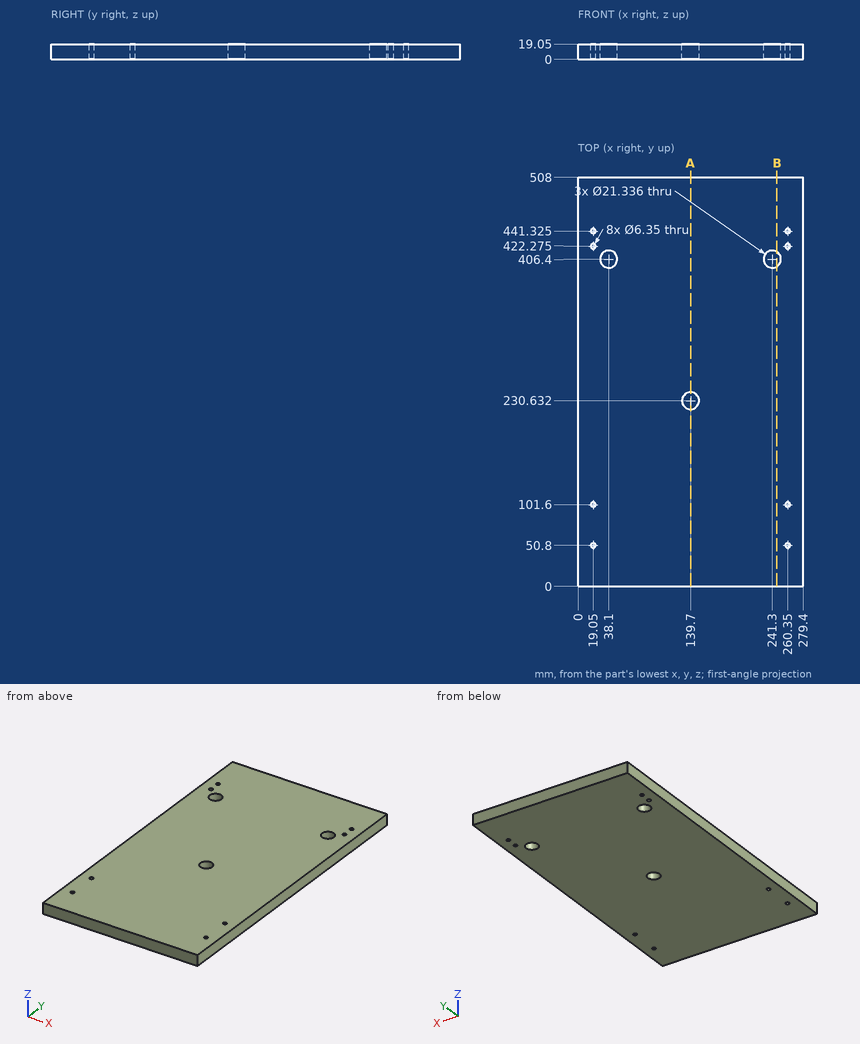
Part print with two shaded views. Sizes in mm from the minimum x, y, z corner. Coordinates: 2 decimals unless noted, no trailing zeros. Write each loop counter-clockwise with the first axis right and the second up, starting at its lowest first coordinate (ties: lowest second). Pieces come first, ordered by that corner, then holes. Notation, with made-up numbers: M 75,15.5 L 108,15.5 A21 ccw 108,51.5 Z; hole C -37,2 d4. An arc over 180 degrees is marked long. Return JSON: item names as keys, results as strings.
Item 1: Slice it at B-B, the plane x = 247. Write the cut outline in (y, z), and give its area (3 significant figures).
Findings below:
{"outline": "M 0,0 L 397.38,0 L 397.38,19.05 L 0,19.05 Z; M 415.42,0 L 508,0 L 508,19.05 L 415.42,19.05 Z", "area": "9,330 mm2"}
Item 2: Slice it at A-A, the plane x = 139.7. Write the cut outline in (y, z), and give its area (3 significant figures).
Findings below:
{"outline": "M 0,0 L 219.96,0 L 219.96,19.05 L 0,19.05 Z; M 241.3,0 L 508,0 L 508,19.05 L 241.3,19.05 Z", "area": "9,270 mm2"}
Item 3: Drop a flat-ended pin along its axis: pin 1 Ø5 at (x, y) = (260.35, 422.275) entering from +Z. Give the stop position or say it passes through.
Findings below:
{"pin 1": "passes through"}
Item 4: Probe line 1 (X direction, y = 101.6, z = 8) (3 decimals); line 2 (X direction, y = 406.4, z = 10.25); line 3 (Y direction, x = 260.35, z = 15) (3 decimals). List the from-to ranges inside material, lowest first. Write a range as from..to.
Findings below:
{"line 1": "x = 0..15.875, 22.225..257.175, 263.525..279.4", "line 2": "x = 0..27.43, 48.77..230.63, 251.97..279.4", "line 3": "y = 0..47.625, 53.975..98.425, 104.775..419.1, 425.45..438.15, 444.5..508"}
